Work out the finished part from the listing and answer in its coordinate system (mm). A direction names the side the tool comes from. Coordinates: 2 decimals unless noted, no trailing zeros. Order: outer loops, then holes, each group sorted by start corner. A loop starts at its lowest first (then second) coordinate and runs counter-clockwise, first axis right, second up. Notation, with made-up numbers: (-3.75, 74.5) -> (48.25, 74.5) arc R21 ccw to (48.25, 101.5) -> close; hole circle Ø6 at (36.25, 70). An arc over 180 degrees is marked (long way). Answer as CSV lines item,"result". Start each with the question number.
Item 1: Section B-B (z = 9.9) is taken. Write down the section's boundary in (x, y), then the cut area to 3 significant figures.
Item 2: Section C-C (x = 23) is taken. Write down the section's boundary in (y, z).
Item 3: Section D-D (y = -28) is taken. Write down the section's boundary in (x, z), then the cut area to 3 significant figures.
Item 4: Section A-A (x = -3.96) is taken. Write down the section's boundary in (y, z).
Item 5: For a pull along Z with two mould halves and no side action, classify faces 6 (the face through (0.168, -1.578, 9.601)), 7 (the face through (46.2, -9, 18)), 8 (the face through (25, -2, 2)), 9 (the face through (41.51, -9.13, 14.92)) as pulls with the +Z half, pulls with the -Z half, needs draft (parallel to the pull), parting line crosses it, or undercut.
Item 6: Which of the six approach directions +Z, -Z, +X, -X, +Y, -Y give full straight-line access (tool end or side, diameter ignored) to faces 1 (the face through (43, -7.9, 10)), 2 (the face through (34.8, -2, 15)), 3 (the face through (37.3, -1.6, 10)), 4 (the face through (0, -24, 10)), 5 (the face through (39.7, -24, 10))?
Item 7: Straight lines are drawn through the part: L1, parallel to Z at x = -3.96, y = -9.7; L2, parallel to Z at x = -3, y = -9; L3, parallel to X at y = -15.5, z = 17.75. For each, find the intervals that lie inside material, in ascending order.
Item 8: Each of these flat-tipped pins is pushed along its axis until it touches: pin 1 Ø8 at (x, z) = (33, 12) entering from +Y; pin 2 Ø5 at (y, z) = (-12, 15.5) entering from -X; pin 3 Ø5 at (x, z) = (-3.5, 11) entering from -Y; pin 4 Ø2 at (x, z) = (-4.5, 9.5) entering from +Y. Where does it stop, or does it pass through?
Autodesk Inventor part; units mm, degrees
ref_plane "YZ Plane" through (0, 0, 0) normal (1, 0, 0) x (0, 1, 0)
ref_plane "XZ Plane" through (0, 0, 0) normal (0, 1, 0) x (-1, 0, 0)
ref_plane "XY Plane" through (0, 0, 0) normal (0, 0, 1) x (1, 0, 0)
sketch "Sketch1" plane through (0, 0, 0) normal (0, 0, 1) x (1, 0, 0)
  line L0 (0, 0) -> (39.7, 0)
  line L1 (39.7, 0) -> (39.7, -37)
  line L2 (39.7, -37) -> (0, -37)
  line L3 (0, -37) -> (0, 0)
  dimension "d0" = 39.7
  dimension "d1" = 37
extrude "Extrusion1" add sketch "Sketch1" along normal blind 19.8
sketch "Sketch2" plane through (39.7, -37, 0) normal (1, 0, 0) x (0, 0, -1)
  line L0 (-19.8, 37) -> (-19.8, 0)
  line L1 (0, 37) -> (0, 0)
  line L2 (0, 37) -> (-19.8, 37)
  line L3 (-19.8, 29.1) -> (0, 29.1)
  line L4 (0, 29.1) -> (0, 26.6)
  line L5 (0, 26.6) -> (-19.8, 26.6)
  line L6 (-19.8, 26.6) -> (-19.8, 29.1)
  dimension "d4" = 2.5
  dimension "d5" = 10.4
extrude "Extrusion2" add sketch "Sketch2" along normal blind 6.5 contours L3 L1 L5 L0
sketch "Sketch3" plane through (39.7, -7.9, 19.8) normal (0, 1, 0) x (1, 0, 0)
  line L0 (6.5, 0) -> (6.5, 19.8)
  arc A0 (5.744, 16.2) -> (5.744, 13.8) centre (3.96, 15) ccw
  arc A1 (5.744, 6) -> (5.744, 3.6) centre (3.96, 4.8) ccw
  line L1 (6.5, 4.8) -> (6.5, 6)
  line L2 (6.5, 6) -> (5.744, 6)
  line L3 (6.5, 3.6) -> (5.744, 3.6)
  line L4 (6.5, 4.8) -> (6.5, 3.6)
  line L5 (6.5, 15) -> (6.5, 13.8)
  line L6 (6.5, 13.8) -> (5.744, 13.8)
  line L7 (5.744, 16.2) -> (6.5, 16.2)
  line L8 (6.5, 16.2) -> (6.5, 15)
  point P0 (-39.7, 19.8)
extrude "Extrusion3" cut sketch "Sketch3" against normal blind 6.5
sketch "Sketch4" plane through (0, -37, 0) normal (-1, 0, 0) x (0, 0, 1)
  line L0 (19.8, 0) -> (19.8, 37)
  line L1 (0, 37) -> (19.8, 37)
  line L2 (0, 0) -> (0, 37)
  line L3 (0, 29.1) -> (19.8, 29.1)
  line L4 (19.8, 29.1) -> (19.8, 26.6)
  line L5 (19.8, 26.6) -> (0, 26.6)
  line L6 (0, 26.6) -> (0, 29.1)
  dimension "d18" = 2.5
  dimension "d19" = 10.4
extrude "Extrusion4" add sketch "Sketch4" along normal blind 6.5 contours L5 L2 L3 L0
sketch "Sketch5" plane through (0, -7.9, 19.8) normal (0, 1, 0) x (1, 0, 0)
  line L0 (-6.5, 19.8) -> (-6.5, 0)
  arc A0 (-5.744, 3.6) -> (-5.744, 6) centre (-3.96, 4.8) ccw
  arc A1 (-5.744, 13.8) -> (-5.744, 16.2) centre (-3.96, 15) ccw
  line L1 (-6.5, 15) -> (-6.5, 16.2)
  line L2 (-6.5, 16.2) -> (-5.744, 16.2)
  line L3 (-5.744, 13.8) -> (-6.5, 13.8)
  line L4 (-6.5, 13.8) -> (-6.5, 15)
  line L5 (-6.5, 4.8) -> (-6.5, 6)
  line L6 (-6.5, 6) -> (-5.744, 6)
  line L7 (-5.744, 3.6) -> (-6.5, 3.6)
  line L8 (-6.5, 3.6) -> (-6.5, 4.8)
  dimension "d25" = 4.3
  dimension "d26" = 1.2
  dimension "d27" = 2.4
extrude "Extrusion5" cut sketch "Sketch5" against normal blind 6.5
sketch "Sketch6" plane through (0, 0, 0) normal (0, 1, 0) x (1, 0, 0)
  line L0 (0, 0) -> (39.7, 0)
  line L1 (0, 0) -> (0, -19.8)
  circle A0 centre (9.9, -9.9) radius 2.5
  dimension "d30" = 5
  dimension "d31" = 19.8
  dimension "d32" = 9.9
  dimension "d33" = 9.9
extrude "Extrusion6" add sketch "Sketch6" along normal blind 3.3
sketch "Sketch7" plane through (0, 0, 0) normal (0, 1, 0) x (1, 0, 0)
  circle A0 centre (9.9, -9.9) radius 2.5
  line L0 (0, -19.8) -> (39.7, -19.8)
  line L1 (39.7, 0) -> (39.7, -19.8)
  line L2 (0, 0) -> (39.7, 0)
  line L3 (0, 0) -> (0, -19.8)
  arc A1 (15.5921, -2) -> (15.5921, -17.8) centre (9.9, -9.9) ccw
  line L4 (34.8, -2) -> (15.5921, -2)
  line L5 (34.8, -17.8) -> (15.5921, -17.8)
  arc A2 (34.8, -12.4) -> (34.8, -7.4) centre (34.8, -9.9) ccw
  line L6 (34.8, -2) -> (34.8, -7.4)
  line L7 (34.8, -12.4) -> (34.8, -17.8)
  dimension "d36" = 2
  dimension "d37" = 2
  dimension "d39" = 5
extrude "Extrusion7" cut sketch "Sketch7" against normal blind 3.2 contours L3 L2 L1 L0
properties part number "7955"
Checked values:
1,outline,"(-6.5, -10.4) -> (0, -10.4) -> (0, -37) -> (39.7, -37) -> (39.7, -10.4) -> (46.2, -10.4) -> (46.2, -7.9) -> (39.7, -7.9) -> (39.7, -3.2) -> (37.3, -3.2) -> (37.3, 0) -> (12.4, 0) -> (12.4, 3.3) -> (7.4, 3.3) -> (7.4, 0) -> (0.16, 0) -> (0.16, -3.2) -> (0, -3.2) -> (0, -7.9) -> (-6.5, -7.9) -> close"
1,area,"1,510 mm^2"
2,outline,"(-37, 0) -> (-3.2, 0) -> (-3.2, 2) -> (0, 2) -> (0, 17.8) -> (-3.2, 17.8) -> (-3.2, 19.8) -> (-37, 19.8) -> close"
3,outline,"(0, 0) -> (39.7, 0) -> (39.7, 19.8) -> (0, 19.8) -> close"
3,area,"786 mm^2"
4,outline,"(-10.4, 0) -> (-7.9, 0) -> (-7.9, 2.65) -> (-10.4, 2.65) -> close; (-10.4, 6.95) -> (-7.9, 6.95) -> (-7.9, 12.85) -> (-10.4, 12.85) -> close; (-10.4, 17.15) -> (-7.9, 17.15) -> (-7.9, 19.8) -> (-10.4, 19.8) -> close"
5,face 6,"parting line crosses it"
5,face 7,"needs draft"
5,face 8,"pulls with the -Z half"
5,face 9,"undercut"
6,face 1,"+Z, -Z, +X, +Y"
6,face 2,"+Z, +X, +Y"
6,face 3,"+X, +Y"
6,face 4,"+Z, -Z, -X, -Y"
6,face 5,"+Z, -Z, +X, -Y"
7,L1,"z = 0 to 2.65, 6.95 to 12.85, 17.15 to 19.8"
7,L2,"z = 0 to 2.88, 6.72 to 13.08, 16.92 to 19.8"
7,L3,"x = 0 to 39.7"
8,pin 1,"stops at y = 0"
8,pin 2,"stops at x = -6.5"
8,pin 3,"stops at y = -10.4"
8,pin 4,"stops at y = -7.9"
